The listing builds one solid part. Answer for the finished solid, in the listing's coordinates (mm). Round coordinates to 2 decimals unless told otherwise and drop trailing zeros. Write each loop counter-clockwise with the first axis right and the second up, starting at its lowest first coordinate (ties: lowest second). Pieces come first, ordered by that corner, then holes.
from build123d import *

# Parameters (mm, degrees)
F1_DEPTH = 18
F3_DEPTH = 18


with BuildPart() as f1:
    # F0 (on Front) → F1 (new body)
    with BuildSketch(Plane.XZ):
        Polygon((333, -435), (333, 435), (-315, 435), (-315, 375), (-333, 375), (-333, -435), align=None)
    extrude(amount=F1_DEPTH)

    # F2 (on face) → F3 (cut)
    with BuildSketch(Plane.XZ.offset(18)):
        with BuildLine():
            Line((333, 340), (278.80919, 340))
            ThreePointArc((278.80919, 340), (203.80919, 265), (278.80919, 190))
            Line((278.80919, 190), (333, 190))
            Line((333, 190), (333, 340))
        make_face()
    extrude(amount=-F3_DEPTH, mode=Mode.SUBTRACT)


solid = f1.part
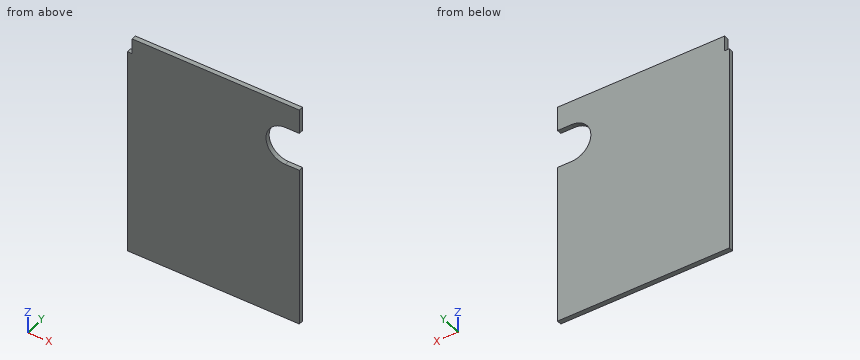
1. Section B-B on z = 265 is taken. Determine the outline of the cut face in (x, y), plus the area to 3 significant figures.
Geometry says:
outline: (-333, -18) - (203.81, -18) - (203.81, 0) - (-333, 0) - close
area: 9,660 mm2
2. Straight lines are drawn through the part: line 1 along Z through (x, y) = (306.5, -1); line 2 along Z through (x, y) = (220.5, -14.25); line 3 along X through (y, z) = (-6.25, 327.5). For each, find the intervals that lie inside material, in ascending order.
Geometry says:
line 1: z = -435 to 190, 340 to 435
line 2: z = -435 to 217.83, 312.17 to 435
line 3: x = -333 to 237.35
3. Section A-A on y = -12.5 is taken. Determine the outline of the cut face in (x, z), plus the area to 3 significant figures.
Geometry says:
outline: (-333, -435) - (333, -435) - (333, 190) - (278.81, 190) arc R75 cw to (278.81, 340) - (333, 340) - (333, 435) - (-315, 435) - (-315, 375) - (-333, 375) - close
area: 561,000 mm2
4. Given pin 1 (5.5 mm diameter, centred on x = -321, y = -10.5, fed in from +Z); pin 2 (9 mm diameter, centred on y = -7, z = 415, fed in from -X), each flat-ended and moving along its own axis, determine where each tip first touches the part or whether it passes through.
Geometry says:
pin 1: stops at z = 375
pin 2: stops at x = -315
